```python
from build123d import *

# Parameters (mm, degrees)
BOSS_EXTRUDE1_DEPTH   = 20
FILLET1_R             = 2
F_4_0MM_DOWEL_HOLE1_D = 4
F_4_0MM_DOWEL_HOLE2_D = 4


with BuildPart() as part:
    # Sketch1 → Boss-Extrude1 (new body)
    with BuildSketch(Plane.XY):
        Polygon((20, 3), (3, 3), (3, 20), (0, 20), (0, 3), (0, 0), (3, 0), (20, 0), align=None)
    extrude(amount=BOSS_EXTRUDE1_DEPTH)

    # Fillet1
    fillet1_edges = [part.edges().sort_by_distance(p)[0] for p in [
        (3, 3, 10),
    ]]
    fillet(fillet1_edges, radius=FILLET1_R)

    # Ø4.0mm Dowel Hole1 (through all)
    with Locations(Plane(origin=(3, 0, 0), x_dir=(0, 0, -1), z_dir=(1, 0, 0))):
        with Locations((-10, 12)):
            Hole(F_4_0MM_DOWEL_HOLE1_D / 2)

    # Ø4.0mm Dowel Hole2 (through all)
    with Locations(Plane(origin=(0, 3, 0), x_dir=(1, 0, 0), z_dir=(0, 1, 0))):
        with Locations((12, -10)):
            Hole(F_4_0MM_DOWEL_HOLE2_D / 2)


solid = part.part
```
Verification items for the finished model (mm, model axes). A direction names the side the tool comes from. Round coordinates to 2 decimals unless told otherwise and drop trailing zeros. Order: outer loops, then holes, each group sorted by start corner. A loop starts at its lowest first (then second) coordinate and runs counter-clockwise, first axis right, second up. Notation, with made-up numbers: (-21, -27) -> (-14, -27) arc R19 cw to (-14, -7) -> close; hole circle Ø1 at (45.25, 76.25). An arc over 180 degrees is marked (long way). Put each result on its own line as item: value. Start each with the question number.
(1) Section check C-C (z = 10). Enter the section's corners in (x, y), then the cut area to 3 significant figures.
(2) Section check D-D (z = 7). Enter the section's corners in (x, y).
(3) Material ranges on line 1 along Y through (x, z) = (0.7, 10); line 2 along X through (y, z) = (13.75, 8.5), recorded low to high.
(4) Section check A-A (y = 12). Enter the section's corners in (x, z).
(5) Depth check by flat-ended pin: pin 1 Ø4.5 at (x, z) = (12, 10) entering from +Y; pin 2 Ø5 at (x, y) = (15, 6.5) entering from -Z; pin 3 Ø6.5 at (y, z) = (12, 10) entering from +X. Enter the tip coordinate at first touch or a pass-through.
(6) Draft check along Z on faces 1 (the face through (1, 14, 10)), 2 (the face through (2.5, 6.3, 20)), 3 (the face through (3, 12.4, 7.6)). Enter one of: +Z half, -Z half, draft (parallel to the pull), parting line (faces both ways), or undercut.
(7) Tool access check on faces 4 (the face through (2.5, 6.3, 0)), 5 (the face through (14.3, 3, 9.9)). Record the directions out of +Z, -Z, +X, -X, +Y, -Y that give a thin tool (end or side, any length) a straight path to the whole face; none if there is none.
Completed:
1. outline: (0, 0) -> (10, 0) -> (10, 3) -> (5, 3) arc R2 cw to (3, 5) -> (3, 10) -> (0, 10) -> close; (0, 14) -> (3, 14) -> (3, 20) -> (0, 20) -> close; (14, 0) -> (20, 0) -> (20, 3) -> (14, 3) -> close
1. area: 87.9 mm2
2. outline: (0, 0) -> (20, 0) -> (20, 3) -> (5, 3) arc R2 cw to (3, 5) -> (3, 20) -> (0, 20) -> close
3. line 1: y = 0 to 10, 14 to 20
3. line 2: x = 0 to 3
4. outline: (0, 0) -> (3, 0) -> (3, 8) -> (0, 8) -> close; (0, 12) -> (3, 12) -> (3, 20) -> (0, 20) -> close
5. pin 1: stops at y = 3
5. pin 2: passes through
5. pin 3: stops at x = 3
6. face 1: undercut
6. face 2: +Z half
6. face 3: draft
7. face 4: -Z, +X, -X, +Y, -Y
7. face 5: +Z, -Z, +X, +Y
